The drawing under review shows one solid part. Ordinate dimensions are in mm from its lowest x, y, z. A direction names the side the tool comes from. Give positions to 0.01 mm unless a question says otherwise; leave off trailing zeros. Order: outer loops, then holes, each group sorted by start corner. A loop starts at its lowest first (then second) coordinate and runs counter-clockwise, first axis right, second up. Notation, with made-up numbers: (80, 23) - (108, 23) arc R17 cw to (108, 48) - close; hole circle Ø11 at (3.25, 73). An arc over 180 degrees is marked (long way). Use CSV: the item, a comma, the result in double quotes. Start each with the question number.
1. Take a section at C-C, the plane x = 48.5. State the section outline as (y, z) points, then the cut area to 3 significant figures.
2. Take a section at B-B, the plane y = 27.75. State the section outline as (x, z) points.
3. Take a section at D-D, the plane y = 11. State the section outline as (x, z) points.
4. For pin 1 (11 mm diameter, centred on y = 24.5, z = 3, fed in from +X); pin 2 (3 mm diameter, centred on x = 26, y = 16, fed in from +Z); pin 3 (3 mm diameter, centred on x = 36.5, z = 17, fed in from +Y), all flat-tipped, find the tip position at first contact; note any pin that passes through.
5. Machinability: for the marked faces 1, 2, 3, 4 and 5, which of the approach directions +Z, -Z, +X, -X, +Y, -Y give a long, thin tool a straight path to every point of the face, cutting with its end or side? Answer none if there is none.
6. Draft analysis for pull direction X (two halves, no side actions). For the marked faces 6, 7 and 8, state which applies: released by +X, released by -X, zero draft, split by the parting line, or undercut.
7. To check wall thickness, follow line 1 (Z direction, x = 3, y = 0.65); line 2 (Y direction, x = 86, z = 5.75); line 3 (X direction, y = 22.25, z = 4.75). State the ranges of each line that lie inside material, in increasing order. Write a range as [from, to].
8. Take a section at A-A, the plane x = 20. State the section outline as (y, z) points, then the cut area to 3 significant figures.
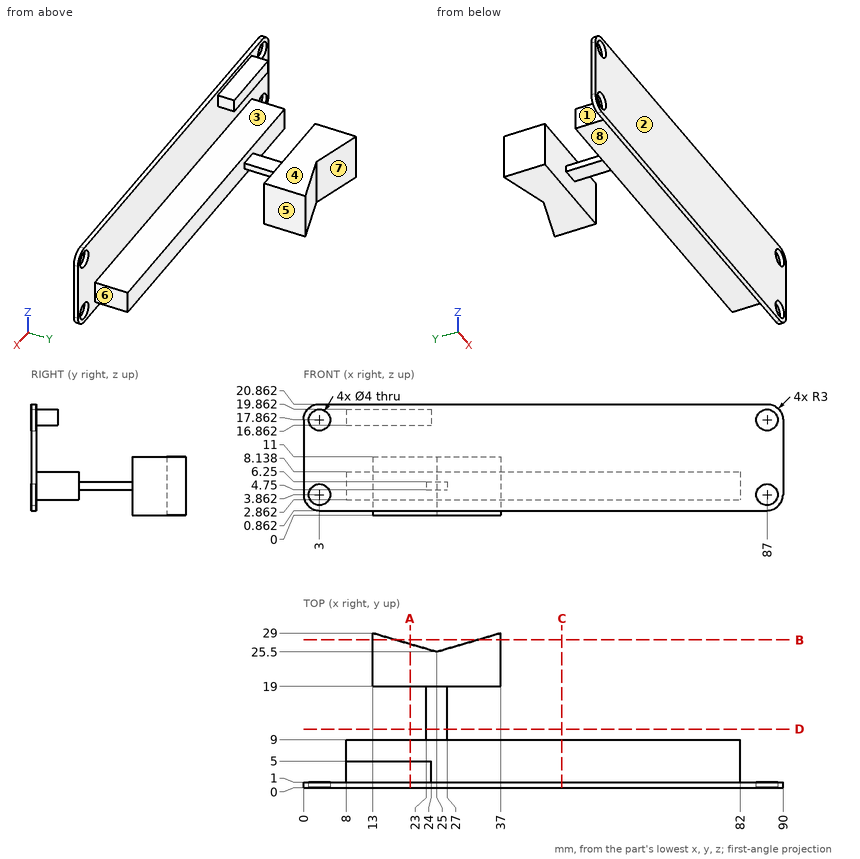
Determined:
1,outline,"(0, 0.86) - (1, 0.86) - (1, 2.86) - (9, 2.86) - (9, 8.14) - (1, 8.14) - (1, 20.86) - (0, 20.86) - close"
1,area,"62.2 mm²"
2,outline,"(13, 0) - (17.29, 0) - (17.29, 11) - (13, 11) - close; (32.71, 0) - (37, 0) - (37, 11) - (32.71, 11) - close"
3,outline,"(23, 4.75) - (27, 4.75) - (27, 6.25) - (23, 6.25) - close"
4,pin 1,"stops at x = 37"
4,pin 2,"stops at z = 6.25"
4,pin 3,"stops at y = 1"
5,face 1,"+Z, -Z, -X, +Y"
5,face 2,"+Z, -Z, +X, -X, -Y"
5,face 3,"+X, -X"
5,face 4,"+Z, +X, -X, +Y"
5,face 5,"+Z, -Z, +X, +Y"
6,face 6,"released by +X"
6,face 7,"undercut"
6,face 8,"zero draft"
7,line 1,"z = [0.86, 1.86], [5.86, 15.86], [19.86, 20.86]"
7,line 2,"y = [0, 1]"
7,line 3,"x = [13, 37]"
8,outline,"(0, 0.86) - (1, 0.86) - (1, 2.86) - (9, 2.86) - (9, 8.14) - (1, 8.14) - (1, 16.86) - (5, 16.86) - (5, 19.86) - (1, 19.86) - (1, 20.86) - (0, 20.86) - close; (19, 0) - (26.96, 0) - (26.96, 11) - (19, 11) - close"
8,area,"162 mm²"
